```python
from build123d import *

# Parameters (mm, degrees)
CIRPATTERN1_COUNT = 12


with BuildPart() as part:
    # Model → Revolve1 (revolve)
    with BuildSketch(Plane.XY, mode=Mode.PRIVATE) as revolve1_sk:
        with BuildLine():
            Line((0, 55.140272), (23.150958, 55.140272))
            ThreePointArc((23.150958, 55.140272), (60.421138671, 50.233559208), (95.151418, 35.847806))
            Line((95.151418, 35.847806), (128.566947896, 16.55534082))
            ThreePointArc((128.566947896, 16.55534082), (133.553991718, 14.489639839), (138.905748896, 13.78506782))
            ThreePointArc((138.905748896, 13.78506782), (139.768990342, 13.856305516), (140.608875713, 14.068091181))
            add(Edge.make_bspline(
                [(140.608875713, 14.068091181), (181.460140896, 28.03089782), (185.649173896, 29.31027082)],
                knots=[0, 0, 0, 1, 1, 1], degree=2))
            Line((185.649173896, 29.31027082), (185.649173896, 76.200272))
            Line((185.649173896, 76.200272), (0, 76.200272))
            Line((0, 76.200272), (0, 55.140272))
        make_face()
    revolve(revolve1_sk.sketch.rotate(Axis((0, 0, 0), (1, 0, 0)), 90), axis=Axis((0, 0, 0), (1, 0, 0)))

    # Sketch3 → #21 (0.159) Diameter Hole1 (revolve, cut)
    with BuildSketch(Plane(origin=(0, 0, 69), x_dir=(0, 0, 1), z_dir=(0, 1, 0))):
        Polygon((0, 0), (0, 26.213317848), (2.0193, 25), (2.0193, 0), align=None)
    f_21_0_159_diameter_hole1 = revolve(axis=Axis((-6.35, 0, 69), (1, 0, 0)), mode=Mode.SUBTRACT)

    # CirPattern1: #21 (0.159) Diameter Hole1 ×12 about axis
    cirpattern1_axis = Axis((0, 0, 0), (1, 0, 0))
    for i in range(1, CIRPATTERN1_COUNT):
        add(f_21_0_159_diameter_hole1.rotate(cirpattern1_axis, i * 360 / CIRPATTERN1_COUNT), mode=Mode.SUBTRACT)


solid = part.part
```
The listing builds one solid part. Answer for the finished solid, in the listing's coordinates (mm). A direction names the side the tool comes from. Round coordinates to 2 decimals unless told otherwise and drop trailing zeros. Order: outer loops, then holes, each group sorted by start corner. A loop starts at its lowest first (then second) coordinate and runs counter-clockwise, first axis right, second up. Notation, with made-up numbers: (89.5, 55.5) - (137.5, 55.5) arc R24 ccw to (137.5, 74.5) - close; hole circle Ø10 at (74, 20). An arc over 180 degrees is marked (long way). Put each result on its own line as item: value. Start each with the question number.
(1) Determine the mould class of faces 1 (the cylindrical face through (91.53, -22.89, 72.68)), 2 (the conical face through (123.23, -5.9, 18.73)), 3 (the flat face through (0, -22.9, 50.4)) for opening direction Z: released by +Z, released by -Z, zero draft, split by the parting line, or undercut.
(2) Given P1, Ø5, axis at x = 51.5, z = 37.5, coming from the +Y side; P2, Ø1, axis at x = 80, z = -18, coming from the +Y side; P3, Ø2.5, axis at y = 34.5, z = -59.76, coming from the -X side, each flat-ended and moving along its own axis, determine where each tip first touches the part or whether it passes through.
(3) Straight lines are drawn through the part: probe 1 along Z at (x, y) = (90.5, -16.5); probe 2 along Z at (x, y) = (84, -31.5); probe 3 along Y at (x, z) = (91.5, -25.5). For each, find the intervals that lie inside material, in ascending order. Write a range as from..to.
(4) Find section A-A (x = 117.5). Give the vertices of the cut face in (y, z).
(5) For faces 4 (the flat face through (185.649, 33, 1)), 5 (the cylindrical face through (11.74, 48.92, 25.44)), determine the directions among +Z, -Z, +X, -X, +Y, -Y from which every point of the face is accessible in a straight line to the end or side of a thin tool.
Reply:
1. face 1: split by the parting line
1. face 2: undercut
1. face 3: zero draft
2. P1: y = 67.69
2. P2: y = 74.16
2. P3: x = 25.46
3. probe 1: -74.39..-34.7, 34.7..74.39
3. probe 2: -69.38..-27.25, 27.25..69.38
3. probe 3: -71.81..-28.02, 28.02..71.81
4. outline: circle Ø152.4 at (0, 0); hole circle Ø45.89 at (0, 0)
5. face 4: +Z, -Z, +X, +Y, -Y
5. face 5: -X
